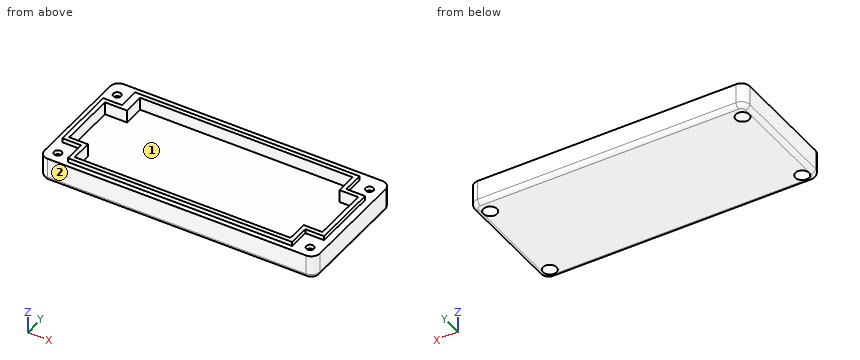
from build123d import *

# Parameters (mm, degrees)
F0_R     = 1.143
F1_DEPTH = 7.112
F2_DEPTH = 8.382
F3_DEPTH = 4.572
F4_R     = 2.032
F5_DEPTH = 5.8674
F6_R     = 1.27


with BuildPart() as f1:
    # F0 (on Top) → F1 (new body)
    with BuildSketch(Plane.XY):
        with BuildLine():
            ThreePointArc((-2.54, 0), (-0.743949, 0.743949), (0, 2.54))
            Line((0, 2.54), (0, 34.29))
            ThreePointArc((0, 34.29), (-0.743949, 36.086051), (-2.54, 36.83))
            Line((-2.54, 36.83), (-79.756, 36.83))
            ThreePointArc((-79.756, 36.83), (-81.552051, 36.086051), (-82.296, 34.29))
            Line((-82.296, 34.29), (-82.296, 2.54))
            ThreePointArc((-82.296, 2.54), (-81.552051, 0.743949), (-79.756, 0))
            Line((-79.756, 0), (-2.54, 0))
        make_face()
        with Locations((-78.867, 3.429)):
            Circle(F0_R, mode=Mode.SUBTRACT)
        with Locations((-3.429, 3.429)):
            Circle(F0_R, mode=Mode.SUBTRACT)
        Polygon((-7.62, 7.874), (-7.62, 1.524), (-74.676, 1.524), (-74.676, 7.874), (-80.264, 7.874), (-80.264, 27.686), (-74.676, 27.686), (-74.676, 34.036), (-7.62, 34.036), (-7.62, 27.686), (-2.032, 27.686), (-2.032, 7.874), align=None, mode=Mode.SUBTRACT)
        with Locations((-78.867, 32.131)):
            Circle(F0_R, mode=Mode.SUBTRACT)
        with Locations((-3.429, 32.131)):
            Circle(F0_R, mode=Mode.SUBTRACT)
    extrude(amount=F1_DEPTH)

    # F0 (on Top) → F2 (join)
    with BuildSketch(Plane.XY):
        Polygon((-74.676, 1.524), (-7.62, 1.524), (-7.62, 7.874), (-2.032, 7.874), (-2.032, 27.686), (-7.62, 27.686), (-7.62, 34.036), (-74.676, 34.036), (-74.676, 27.686), (-80.264, 27.686), (-80.264, 7.874), (-74.676, 7.874), align=None)
        Polygon((-8.89, 9.144), (-8.89, 2.794), (-73.406, 2.794), (-73.406, 9.144), (-78.994, 9.144), (-78.994, 26.416), (-72.402207, 26.416), (-72.402207, 32.766), (-8.89, 32.766), (-8.89, 26.416), (-3.302, 26.416), (-3.302, 9.144), align=None, mode=Mode.SUBTRACT)
    extrude(amount=F2_DEPTH)

    # F0 (on Top) → F3 (join)
    with BuildSketch(Plane.XY):
        Polygon((-73.406, 2.794), (-8.89, 2.794), (-8.89, 9.144), (-3.302, 9.144), (-3.302, 26.416), (-8.89, 26.416), (-8.89, 32.766), (-72.402207, 32.766), (-72.402207, 26.416), (-78.994, 26.416), (-78.994, 9.144), (-73.406, 9.144), align=None)
    extrude(amount=F3_DEPTH)

    # F4 (on face) → F5 (cut)
    with BuildSketch(Plane.XY):
        with Locations((-3.429, 32.258)):
            Circle(F4_R)
        with Locations((-78.871086, 32.258)):
            Circle(F4_R)
        with Locations((-3.429, 3.429)):
            Circle(F4_R)
        with Locations((-78.867, 3.429)):
            Circle(F4_R)
    extrude(amount=F5_DEPTH, mode=Mode.SUBTRACT)

    # F6
    f6_edges = [f1.edges().sort_by_distance(p)[0] for p in [
        (-41.148, 36.83, 0),
    ]]
    fillet(f6_edges, radius=F6_R)


solid = f1.part
Source: CAD feature listing. Evaluate the final solid. Frame: model axes, mm. Face numbers are marked on the shaded views. Coordinates: 2 decimals unless noted, no trailing zeros. Loops run counter-clockwise (first coordinate to the right, second up) from the corner with the lowest first, then second, coordinate; pieces in that order, holes last. Notation, with made-up numbers: M 2,68.25 L 41,68.25 A7 cw 41,74.25 Z; hole C 15.25,13 d10. An arc over 180 degrees is marked long. Answer in a Markdown table with one row per item.
Q1. Section A-A on x = -45.5. Return the cut outline in (y, z).
Answers below:
| item | result |
|---|---|
| outline | M 0,1.27 A1.27 ccw 1.27,0 L 35.56,0 A1.27 ccw 36.83,1.27 L 36.83,7.11 L 34.04,7.11 L 34.04,8.38 L 32.77,8.38 L 32.77,4.57 L 2.79,4.57 L 2.79,8.38 L 1.52,8.38 L 1.52,7.11 L 0,7.11 Z |
Q2. Section B-B on y = 13. Return the cut outline in (x, z), plus the area to 3 significant figures.
Answers below:
| item | result |
|---|---|
| outline | M -82.3,1.27 A1.27 ccw -81.03,0 L -1.27,0 A1.27 ccw 0,1.27 L 0,7.11 L -2.03,7.11 L -2.03,8.38 L -3.3,8.38 L -3.3,4.57 L -78.99,4.57 L -78.99,8.38 L -80.26,8.38 L -80.26,7.11 L -82.3,7.11 Z |
| area | 396 mm^2 |
Q3. Draft query along X for the marked faces 1 and 2. Return one class per face: pulls with the +X half, pulls with the -X half, needs draft (parallel to the pull), parting line crosses it, or undercut.
Answers below:
| item | result |
|---|---|
| face 1 | undercut |
| face 2 | needs draft |
Q4. Ray query, probe 1 along X at (y, z) = (25, 7); probe 2 along Y at (x, z) = (-63.5, 5); probe 3 along X at (y, z) = (30.5, 0.75). Return the intervals inside material, ascending. Write a range as from..to.
Answers below:
| item | result |
|---|---|
| probe 1 | x = -82.3..-78.99, -3.3..0 |
| probe 2 | y = 0..2.79, 32.77..36.83 |
| probe 3 | x = -82.18..-79.89, -77.85..-4.45, -2.41..-0.11 |
Q5. First-contact query: pin 1 (5.5 mm diameter, centred on x = -78.867, y = 3.429, fed in from +Z); pin 2 (5 mm diameter, centred on x = -34.5, y = 20.5, fed in from +Z); pin 3 (1.4 mm diameter, centred on x = -6, z = 8, fed in from -Y); pin 4 (12 mm diameter, centred on x = -55, y = 28.5, fed in from -Z). Flat tips, straight axial feed; report the tip coordinate or a pass-through.
Answers below:
| item | result |
|---|---|
| pin 1 | stops at z = 7.11 |
| pin 2 | stops at z = 4.57 |
| pin 3 | stops at y = 7.87 |
| pin 4 | stops at z = 0 |
